Read the model definition and answer for the solid it produces. Units are mm, in the model's axes. Face numbers are marked on the shaded views. A direction names the side the tool comes from. Give positions to 0.01 mm unless a question says otherwise; leave off trailing zeros. Loops run counter-clockwise (first coordinate to the right, second up) from the corner with the lowest first, then second, coordinate; pieces in that order, holes last. Notation, with made-up numbers: M 76.25,19.5 L 131.25,19.5 A21 cw 131.25,36.5 Z; hole C -13.5,29 d1. An arc over 180 degrees is marked long. Return JSON: item names as keys, results as strings. Group by question number.
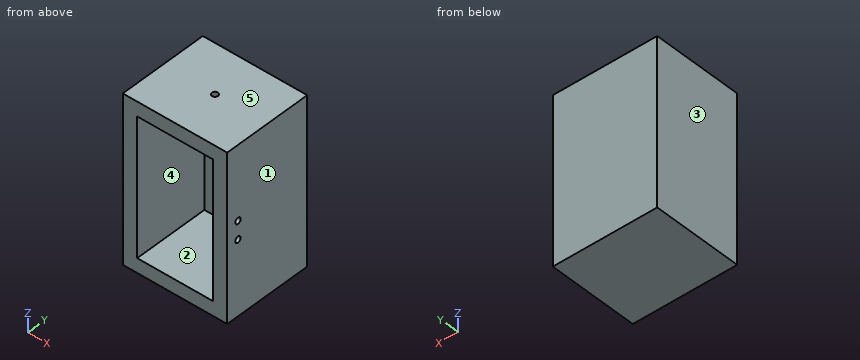
```python
from build123d import *

# Parameters (mm, degrees)
F2_DEPTH      = 140
F2_DEPTH_BACK = 80
F3_W          = 100
F3_H          = 19.05
F4_DEPTH      = 100
F5_R          = 4
F6_DEPTH      = 19.05
F7_R          = 4
F8_DEPTH      = 20


with BuildPart() as f2:
    # F1 (on offset) → F2 (new body, two sides)
    with BuildSketch(Plane.XY.offset(-5.5)) as f2_sk:
        Polygon((-55.145783, -50), (-55.145783, 50), (44.854217, 50), (44.854217, -50), (63.904217, -50), (63.904217, 69.05), (-74.195783, 69.05), (-74.195783, -50), align=None)
    extrude(amount=F2_DEPTH)
    extrude(f2_sk.sketch, amount=-F2_DEPTH_BACK)

    # F3 (on face) → F4 (join)
    with BuildSketch(Plane.XZ.offset(-50)):
        with Locations((-5.145783, 124.975)):
            Rectangle(F3_W, F3_H)
        with Locations((-5.145783, -75.975)):
            Rectangle(F3_W, F3_H)
    extrude(amount=F4_DEPTH)

    # F5 (on face) → F6 (cut)
    with BuildSketch(Plane.XY.offset(134.5)):
        with Locations((-5.145783, 9.525)):
            Circle(F5_R)
    extrude(amount=-F6_DEPTH, mode=Mode.SUBTRACT)

    # F7 (on face) → F8 (cut)
    with BuildSketch(Plane.YZ.offset(63.904217)):
        with Locations((-34, 13)):
            Circle(F7_R)
        with Locations((-34, 37)):
            Circle(F7_R)
    extrude(amount=-F8_DEPTH, mode=Mode.SUBTRACT)


solid = f2.part
```
1. Find section C-C (y = -34). Write down the section's boundary in (x, z), and give its area (3 significant figures).
2. Find section A-A (z = 37). Write down the section's boundary in (x, y).
3. Find section B-B (y = -18.5). Write down the section's boundary in (x, z).
4. Flat-ended cylindrical pins translate along their axes: P1, Ø7, axis at y = -34, z = 37, coming from the +X side; P2, Ø12, axis at x = 19.5, z = 37.5, coming from the -Y side. Find the tip coordinate at first contact, or state that the pin passes through.
5. Find section D-D (x = 14). Write down the section's boundary in (y, z).
6. The mould has two halves that part along Z. Classify the marked faces 3, 4 and 5: +Z half, -Z half, draft (parallel to the pull), parting line (faces both ways), or undercut.
7. Straight lines are drawn through the part: line 1 along Z through (x, y) = (55, -34); line 2 along Z through (x, y) = (40, 21); line 3 along X through (y, z) = (22, 24). For each, find the intervals that lie inside material, in ascending order.
8. For the marked faces 1 and 2, determine the directions among +Z, -Z, +X, -X, +Y, -Y from which every point of the face is accessible in a straight line to the end or side of a thin tool.
Result:
{
 "1": {"outline": "M -74.2,-85.5 L 63.9,-85.5 L 63.9,9 L 44.85,9 L 44.85,-66.45 L -55.15,-66.45 L -55.15,115.45 L 44.85,115.45 L 44.85,41 L 63.9,41 L 63.9,134.5 L -74.2,134.5 Z; M 44.85,17 L 63.9,17 L 63.9,33 L 44.85,33 Z", "area": "11,900 mm2"},
 "2": {"outline": "M -74.2,-50 L -55.15,-50 L -55.15,50 L 44.85,50 L 44.85,-30 L 63.9,-30 L 63.9,69.05 L -74.2,69.05 Z; M 44.85,-50 L 63.9,-50 L 63.9,-38 L 44.85,-38 Z"},
 "3": {"outline": "M -74.2,-85.5 L 63.9,-85.5 L 63.9,134.5 L -74.2,134.5 Z; hole M -55.15,-66.45 L 44.85,-66.45 L 44.85,115.45 L -55.15,115.45 Z"},
 "4": {"P1": "stops at x = -55.15", "P2": "stops at y = 50"},
 "5": {"outline": "M -50,-85.5 L 69.05,-85.5 L 69.05,134.5 L -50,134.5 L -50,115.45 L 50,115.45 L 50,-66.45 L -50,-66.45 Z"},
 "6": {"face 3": "draft", "face 4": "undercut", "face 5": "+Z half"},
 "7": {"line 1": "z = -85.5 to 9, 17 to 33, 41 to 134.5", "line 2": "z = -85.5 to -66.45, 115.45 to 134.5", "line 3": "x = -74.2 to -55.15, 44.85 to 63.9"},
 "8": {"face 1": "+Z, -Z, +X, +Y, -Y", "face 2": "-Y"}
}
